Can you work these out from the model? Positions are in its coordinate system, mm. A direction names the side the tool comes from. Coordinates: 2 decimals unless noted, no trailing zeros. Order: outer loops, then holes, each group sorted by start corner. A loop starts at its lowest first (then second) coordinate and runs counter-clockwise, first axis right, second up. Notation, with made-up numbers: (33, 6.25) -> (78, 6.25) arc R18 cw to (78, 31.25) -> close; hole circle Ø6 at (78, -3.5). An arc over 180 degrees is marked (long way). Answer as a JSON object with one key per item and string values. Group by question number.
(1) I want a section at A-A, the plane x = -12.5. List the corners of the cut face in (y, z) for me.
(2) I want a section at B-B, the plane y = -24. List the corners of the cut face in (x, z) for me, plus the area to 3 significant figures.
(3) I want a section at D-D, the plane z = -13. List the corners of the cut face in (x, y) for me.
(4) I need wall thicknesses on line 1 (Z direction, x = -13.75, y = -6); line 2 (Z direction, x = -12, y = -34.5); line 3 (Z direction, x = -10.25, y = 41). Which ranges of each line are inside material? Lowest first, please.
(5) I want a section at C-C, the plane z = 40. List the corners of the cut face in (x, y) for me.
(6) Which directions (+Z, -Z, +X, -X, +Y, -Y) give clear straight access to the entire face, cutting with the end or side of a thin tool? Please do faces 1 (the flat face through (-11, -24, -4.051)), 2 (the cylindrical face through (-11.311, 20.224, 5.892)), 3 (the flat face through (-6.241, 14, -2)), 4 (the cylindrical face through (-8.21, -32.07, 1.52)), 5 (the flat face through (-16.241, 14, -2)).
(7) For pin 1 (1 mm diameter, centred on x = -11.5, y = -15, fed in from -Z); pin 2 (9 mm diameter, centred on y = 35.23, z = 5.95, fed in from -X); pin 3 (3 mm diameter, centred on y = 37, z = 7.5, fed in from +X); pin 4 (5 mm diameter, centred on y = -12.5, z = 19, fed in from -X), each with a flat end and sliding along its axis, tell me the tip position at first contact or that it passes through.
(8) If we mould it in two halves opening along Z, with no side actions, what happens to faces 6 (the cylindrical face through (-11.311, -1.23, -4.842)), 7 (the flat face through (-10.2, 42.9, 30.9)), 8 (the cylindrical face through (-11.17, -43.8, 15.35))? For each: pulls with the +Z half, pulls with the -Z half, needs draft (parallel to the pull), parting line crosses it, or undercut.
from build123d import *

# Parameters (mm, degrees)
SKETCH_W           = 89.59788
SKETCH_H           = 20
PAD_DEPTH          = 10
SKETCH001_W        = 4
SKETCH001_H        = 19
PAD001_DEPTH       = 3
HOLE_D             = 5.5
HOLE_DEPTH         = 25
HOLE_CBORE_D       = 10
HOLE_CBORE_DEPTH   = 4
FILLET_R           = 2
SKETCH003_R        = 3.2
POCKET_DEPTH       = 13.001
SKETCH004_R        = 0.5
PAD002_DEPTH       = 10
POCKET001_DEPTH    = 17.5
FILLET001_R        = 15
POCKET002_DEPTH    = 3
POCKET002_FACE32_W = 4
POCKET002_FACE32_H = 19
POCKET003_DEPTH    = 3


with BuildPart() as part:
    # Sketch (on Face2 of Binder) → Pad (new body)
    with BuildSketch(Plane.YZ.offset(237.459106)):
        with Locations((0.426081, 189.84877)):
            Rectangle(SKETCH_W, SKETCH_H)
        with BuildLine():
            ThreePointArc((-16.372859, 192.857809), (-19.372859, 189.857809), (-16.372859, 186.857809))
            Line((-16.372859, 186.857809), (17.225021, 186.857809))
            ThreePointArc((17.225021, 186.857809), (20.225021, 189.857809), (17.225021, 192.857809))
            Line((-16.372859, 192.857809), (17.225021, 192.857809))
        make_face(mode=Mode.SUBTRACT)
    extrude(amount=PAD_DEPTH)

    # Sketch001 (on Face9 of Pad) → Pad001 (join)
    with BuildSketch(Plane(origin=(237.459106, 0, 0), x_dir=(0, -1, 0), z_dir=(-1, 0, 0))):
        with Locations((-23.225021, 189.84877)):
            Rectangle(SKETCH001_W, SKETCH001_H)
        with Locations((22.372859, 189.857809)):
            Rectangle(SKETCH001_W, SKETCH001_H)
    extrude(amount=PAD001_DEPTH)

    # Hole
    with Locations(Plane.YZ.offset(247.459106)):
        with Locations((-34.372859, 189.857809), (35.225021, 189.84877)):
            CounterBoreHole(HOLE_D / 2, HOLE_CBORE_D / 2, HOLE_CBORE_DEPTH, depth=HOLE_DEPTH)

    # Fillet
    fillet_edges = [part.edges().sort_by_distance(p)[0] for p in [
        (242.459106, 45.225021, 199.84877),
        (242.459106, 45.225021, 179.84877),
        (242.459106, -44.372859, 199.84877),
        (242.459106, -44.372859, 179.84877),
    ]]
    fillet(fillet_edges, radius=FILLET_R)

    # Sketch003 (on Face5 of Fillet) → Pocket (cut, through all)
    with BuildSketch(Plane.YZ.offset(247.459106)):
        with Locations((25.225021, 189.84877)):
            Circle(SKETCH003_R)
    extrude(amount=-POCKET_DEPTH, mode=Mode.SUBTRACT)

    # Sketch004 (on Face5 of Pocket) → Pad002 (join)
    with BuildSketch(Plane.YZ.offset(247.459106)):
        with BuildLine():
            ThreePointArc((52.725021, 220.159659), (47.198029, 229.103495), (36.726581, 228.160829))
            Line((36.726581, 228.160829), (-1.038162, 199.84877))
            Line((43.225021, 199.84877), (-1.038162, 199.84877))
            Line((43.225021, 179.84877), (43.225021, 199.84877))
            Line((-1.038162, 179.84877), (43.225021, 179.84877))
            Line((-1.038162, 179.84877), (36.726581, 151.536712))
            ThreePointArc((36.726581, 151.536712), (47.198029, 150.594045), (52.725021, 159.537881))
            Line((52.725021, 159.537881), (52.725021, 220.159659))
        make_face()
        with Locations((42.725021, 220.159659)):
            Circle(SKETCH004_R, mode=Mode.SUBTRACT)
        with Locations((42.725021, 159.537881)):
            Circle(SKETCH004_R, mode=Mode.SUBTRACT)
    extrude(amount=-PAD002_DEPTH)

    # Sketch005 (on DatumPlane) → Groove (revolve, cut)
    with BuildSketch(Plane(origin=(247.459106, 42.725021, 159.537881), x_dir=(0, 0, 1), z_dir=(0, 1, 0))):
        Polygon((0, 21.851335), (0, -8), (-29.851335, 21.851335), align=None)
    revolve(axis=Axis((247.459106, 42.725021, 159.537881), (1, 0, 0)), mode=Mode.SUBTRACT)

    # Sketch006 (on DatumPlane) → Pocket001 (cut, symmetric)
    with BuildSketch(Plane(origin=(247.459106, 42.725021, 220.159659), x_dir=(0, -0.694658, 0.71934), z_dir=(0, 0.71934, 0.694658))):
        Polygon((0, -8), (12.395839, 4.192451), (-11.9924, 4.192451), align=None)
    extrude(amount=POCKET001_DEPTH, both=True, mode=Mode.SUBTRACT)

    # Fillet001
    fillet001_edges = [part.edges().sort_by_distance(p)[0] for p in [
        (242.459106, -1.038162, 179.84877),
        (242.459106, -1.038162, 199.84877),
    ]]
    fillet(fillet001_edges, radius=FILLET001_R)

    # Fillet001 Face36 → Pocket002 (cut)
    with BuildSketch(Plane(origin=(234.459106, 23.052701, 189.84877), x_dir=(0, 1, 0), z_dir=(-1, 0, 0))):
        with BuildLine():
            Line((2.17232, -9.5), (2.17232, -3.2))
            ThreePointArc((2.17232, -3.2), (-1.02768, 0), (2.17232, 3.2))
            Line((2.17232, 3.2), (2.17232, 9.5))
            Line((2.17232, 9.5), (-1.82768, 9.5))
            Line((-1.82768, 9.5), (-1.82768, -9.5))
            Line((-1.82768, -9.5), (2.17232, -9.5))
        make_face()
    extrude(amount=-POCKET002_DEPTH, mode=Mode.SUBTRACT)

    # Pocket002 Face32 → Pocket003 (cut)
    with BuildSketch(Plane(origin=(234.459106, -22.372859, 189.857809), x_dir=(0, 1, 0), z_dir=(-1, 0, 0))):
        Rectangle(POCKET002_FACE32_W, POCKET002_FACE32_H)
    extrude(amount=-POCKET003_DEPTH, mode=Mode.SUBTRACT)


with BuildPart() as part_1:
    # Body placement: moved
    add(part.part.moved(Location((-253.7, 0, -183.9))))


solid = part_1.part
Computed values:
{
 "1": {"outline": "(-44.37, -2.05) arc R2 ccw to (-42.37, -4.05) -> (-6.04, -4.05) arc R15 cw to (2.96, -7.05) -> (36.73, -32.36) arc R10 ccw to (52.73, -24.36) -> (52.73, 36.26) arc R10 ccw to (51, 41.87) -> (31.33, 22.87) -> (28.91, 25.38) -> (48.58, 44.37) arc R10 ccw to (36.73, 44.26) -> (2.96, 18.95) arc R15 cw to (-6.04, 15.95) -> (-42.37, 15.95) arc R2 ccw to (-44.37, 13.95) -> close; hole circle Ø5.5 at (-34.37, 5.96); hole (-16.37, 2.96) -> (17.23, 2.96) arc R3 ccw to (17.23, 8.96) -> (-16.37, 8.96) arc R3 ccw to start; hole circle Ø6.4 at (25.23, 5.95); hole circle Ø5.5 at (35.23, 5.95); hole circle Ø3.48 at (42.73, -24.36)"},
 "2": {"outline": "(-16.24, -4.05) -> (-6.24, -4.05) -> (-6.24, 15.95) -> (-16.24, 15.95) -> close", "area": "200 mm2"},
 "3": {"outline": "(-16.24, 10.9) -> (-6.24, 10.9) -> (-6.24, 52.73) -> (-16.24, 52.73) -> close"},
 "4": {"line 1": "z = -4.05 to 2.96, 8.96 to 15.95", "line 2": "z = -4.05 to 3.21, 8.7 to 15.95", "line 3": "z = -34.21 to -27.96, -20.76 to 29.14, 40.23 to 46.11"},
 "5": {"outline": "(-16.24, 31.04) -> (-6.24, 31.04) -> (-6.24, 34.89) -> (-14.24, 46.6) -> (-10.43, 52) -> (-16.24, 52) -> close"},
 "6": {"face 1": "-Z, +X, -X, -Y", "face 2": "+X, -X", "face 3": "+Z, -Z, +X, +Y, -Y", "face 4": "+X", "face 5": "+Z, -Z, -X, +Y, -Y"},
 "7": {"pin 1": "stops at z = -4.05", "pin 2": "stops at x = -16.24", "pin 3": "stops at x = -10.24", "pin 4": "passes through"},
 "8": {"face 6": "pulls with the -Z half", "face 7": "undercut", "face 8": "pulls with the +Z half"}
}
